Design review of the part built by this model. Coordinates are the model's own, in mm. A direction names the side the tool comes from. Round coordinates to 2 decimals unless told otherwise and drop trailing zeros. Loops run counter-clockwise (first coordinate to the right, second up) from the corner with the lowest first, then second, coordinate; pieces in that order, holes last. Notation, with made-up numbers: (-15, 20.5) -> (0, 20.5) arc R8 cw to (0, 27.5) -> close; hole circle Ø5 at (-19, 38). An arc over 180 degrees is marked (long way). Answer as CSV lines item,"result". Start each with the question number.
(1) Take a section at D-D, the plane z = -0.7. Write out the cut boundary in (x, y), and give its area (3 significant figures).
(2) Machinability: for faces 1 (the face through (0, 3.2, 2)), 2 (the face through (-5, 3.2, 2)), 3 (the face through (5, 2.6, 2)), 4 (the face through (6.4, 3, -3)), 5 (the face through (0, 2.6, 2)), which of the approach directions +Z, -Z, +X, -X, +Y, -Y give a long, thin tool a straight path to every point of the face, cutting with its end or side? Answer none if there is none.
(3) For P1, Ø0.9, axis at y = 3.5, z = 0.5, coming from the +X side; P2, Ø0.9, axis at x = 0, z = 2, coming from the +Y side; P3, Ø3, axis at x = 0.5, z = -7.5, coming from the -Y side, all flat-tipped, find the tip position at first contact; note any pin that passes through.
(4) Take a section at C-C, the plane x = 1. Write out the cut boundary in (y, z).
(5) Draft analysis for pull direction Z (two halves, no side actions). For faces 6 (the face through (1.7, 1.4, -7.71)), 7 (the face through (0, 3, -5.8)), 8 (the face through (2.07, 2.92, -8.05)), 9 (the face through (1.975, 2.921, -7.616)), state which applies: +Z half, -Z half, draft (parallel to the pull), parting line (faces both ways), or undercut.
(6) Take a section at B-B, the plane y = 4.15. Write out the cut boundary in (x, z) (3 decimals).
(7) Take a section at A-A, the plane z = 3. Write out the cut boundary in (x, y), and give its area (3 significant figures).
(8) To check wall thickness, follow line 1 (X direction, y = 3.1, z = 1.75); line 2 (X direction, y = 1.6, z = -0.7); line 3 (Z direction, x = -4, y = 4.15) (3 decimals). State the ranges of each line that lie inside material, in increasing order. Write a range as from..to.
from build123d import *

# Parameters (mm, degrees)
SKETCH1_R           = 1
BOSS_EXTRUDE1_DEPTH = 5.8
EXTRUDE_THIN1_DEPTH = 1.5
BOSS_EXTRUDE2_DEPTH = 0.3


with BuildPart() as part:
    # Sketch1 → Boss-Extrude1 (new body)
    with BuildSketch(Plane(origin=(0, 0, 0), x_dir=(1, 0, 0), z_dir=(0, 1, 0))):
        Polygon((6.4, 0), (6.4, 5.8), (-6.4, 5.8), (-6.4, 0), (-4.480616855, 0), (-4.480616855, -0.794991669), (-2.082638034, -0.794991669), (-2.082638034, 0), (2.15791372, 0), (2.15791372, -0.794991669), (4.480616855, -0.794991669), (4.480616855, 0), align=None)
        with Locations(Location((3.25, 0.7, 0), (0, 0, 270))):
            Circle(SKETCH1_R, mode=Mode.SUBTRACT)
        with Locations(Location((-3.25, 0.7, 0), (0, 0, 270))):
            Circle(SKETCH1_R, mode=Mode.SUBTRACT)
    extrude(amount=BOSS_EXTRUDE1_DEPTH)

    # Sketch2 → Extrude-Thin1 (add, symmetric)
    with BuildSketch(Plane(origin=(0, 2.9, 0), x_dir=(1, 0, 0), z_dir=(0, 1, 0))):
        with BuildLine():
            Line((8.670419942, 9.598188691), (-4.715076855, 6.45728949))
            ThreePointArc((-4.715076855, 6.45728949), (-5.101788699, 6.233385099), (-5.299071375, 5.832437755))
            Line((-5.299071375, 5.832437755), (-4.904367476, 5.767562245))
            ThreePointArc((-4.904367476, 5.767562245), (-4.80955319, 5.960258009), (-4.623699024, 6.067866722))
            Line((-4.623699024, 6.067866722), (8.761797773, 9.208765923))
            Line((8.761797773, 9.208765923), (8.670419942, 9.598188691))
        make_face()
    extrude(amount=EXTRUDE_THIN1_DEPTH, both=True)

    # Sketch3 → Boss-Extrude2 (add, symmetric)
    with BuildSketch(Plane(origin=(0, 2.9, 0), x_dir=(1, 0, 0), z_dir=(0, 1, 0))):
        with BuildLine():
            Line((-5.579037079, 0), (-5.579037079, -4.131158505))
            ThreePointArc((-5.579037079, -4.131158505), (-5.179037079, -4.531158505), (-4.779037079, -4.131158505))
            Line((-4.779037079, -4.131158505), (-4.779037079, 0))
            Line((-4.779037079, 0), (-5.579037079, 0))
        make_face()
        with BuildLine():
            Line((-0.4, -4.131158505), (-0.4, 0))
            Line((-0.4, 0), (0.4, 0))
            Line((0.4, 0), (0.4, -4.131158505))
            ThreePointArc((0.4, -4.131158505), (0, -4.531158505), (-0.4, -4.131158505))
        make_face()
        with BuildLine():
            Line((4.779037079, 0), (5.579037079, 0))
            Line((5.579037079, 0), (5.579037079, -4.131158505))
            ThreePointArc((5.579037079, -4.131158505), (5.179037079, -4.531158505), (4.779037079, -4.131158505))
            Line((4.779037079, -4.131158505), (4.779037079, 0))
        make_face()
    extrude(amount=BOSS_EXTRUDE2_DEPTH, both=True)


solid = part.part
The answers:
1,outline,"(-6.4, 0) -> (-4.25, 0) -> (-4.25, 5.8) -> (-6.4, 5.8) -> close; (-2.25, 0) -> (2.25, 0) -> (2.25, 5.8) -> (-2.25, 5.8) -> close; (4.25, 0) -> (6.4, 0) -> (6.4, 5.8) -> (4.25, 5.8) -> close"
1,area,"51.0 mm²"
2,face 1,"+Z, +Y"
2,face 2,"+Z, -X, +Y"
2,face 3,"+Z, +X, -Y"
2,face 4,"+Z, +X, +Y, -Y"
2,face 5,"+Z, -Y"
3,P1,"x = 5.58"
3,P2,"y = 3.2"
3,P3,"y = 1.4"
4,outline,"(0, -5.8) -> (5.8, -5.8) -> (5.8, 0) -> (0, 0) -> close; (1.4, -7.8) -> (4.4, -7.8) -> (4.4, -7.39) -> (1.4, -7.39) -> close"
5,face 6,"draft"
5,face 7,"undercut"
5,face 8,"-Z half"
5,face 9,"undercut"
6,outline,"(-6.4, -5.8) -> (-5.102, -5.8) -> (-5.299, -5.832) arc R0.77 ccw to (-4.715, -6.457) -> (8.67, -9.598) -> (8.762, -9.209) -> (-4.624, -6.068) arc R0.37 cw to (-4.898, -5.8) -> (6.4, -5.8) -> (6.4, 0) -> (4.481, 0) -> (4.481, 0.795) -> (2.158, 0.795) -> (2.158, 0) -> (-2.083, 0) -> (-2.083, 0.795) -> (-4.481, 0.795) -> (-4.481, 0) -> (-6.4, 0) -> close; hole circle Ø2 at (-3.25, -0.7); hole circle Ø2 at (3.25, -0.7)"
7,outline,"(-5.58, 2.6) -> (-4.78, 2.6) -> (-4.78, 3.2) -> (-5.58, 3.2) -> close; (-0.4, 2.6) -> (0.4, 2.6) -> (0.4, 3.2) -> (-0.4, 3.2) -> close; (4.78, 2.6) -> (5.58, 2.6) -> (5.58, 3.2) -> (4.78, 3.2) -> close"
7,area,"1.44 mm²"
8,line 1,"-5.58..-4.78, -0.4..0.4, 4.78..5.58"
8,line 2,"-6.4..-4.25, -2.25..2.25, 4.25..6.4"
8,line 3,"-6.625..-6.214, -5.8..-1.361, -0.039..0.795"
